Geometry check sheet. Reference: the model listing, model coordinates, mm. Face numbers are marked on the shaded views. A direction names the side the tool comes from. Round coordinates to 2 decimals unless told otherwise and drop trailing zeros. Order: outer loops, then holes, each group sorted by start corner. A loop starts at its lowest first (then second) coordinate and runs counter-clockwise, first axis right, second up. Notation, with made-up numbers: (22, -39) -> (54, -39) arc R22 ccw to (54, -14) -> close; hole circle Ø1 at (-8.75, 18.25). An arc over 180 degrees is marked (long way). Use a Markdown table: item, result. Add a question column.
Item 1: Set-up check for the marked faces 4 and 5: record each of +Z, -Z, +X, -X, +Y, -Y from which the full face is reachable in a straight line by a thin tool's end or side.
Item 2: Sectioned sample at A-A, the plane z = 0. Record the cut outline in (x, y).
Item 3: Sectioned sample at D-D, the plane z = 17. Record the cut outline in (x, y), and give its area (3 significant figures).
Item 4: Material ranges on probe 1 along X at (y, z) = (9.25, 0); probe 2 along Y at (x, z) = (24, 14); probe 3 along Y at (x, z) = (16, 2.5), recorded low to high. Write a range as [from, to].
Item 5: Sectioned sample at B-B, the plane x = 20. Record the cut outline in (y, z).
Item 6: Mould release check, pull along Z, two halves, no side actions. Record for the marked faces 1, 2 and 3: pulls with the +Z half, pulls with the -Z half, needs draft (parallel to the pull), parting line crosses it, or undercut.
Item 7: Gauge pin test, flat ends, axial feed: pin 1 Ø5 at (x, z) = (22.5, -1.5) entering from +Y; pin 2 Ø6 at (x, z) = (20, 0) entering from +Y. Record the tip position at first contact, or that the pin passes through.
Item 8: Sectioned sample at C-C, the plane y = 26. Record the cut outline in (x, z), and give its area (3 significant figures).
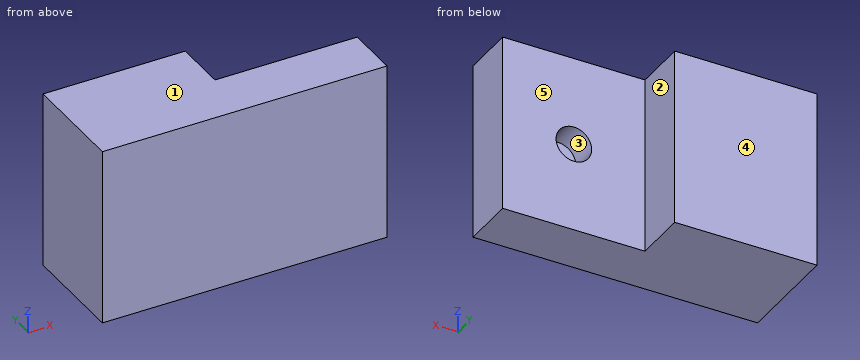
from build123d import *

# Parameters (mm, degrees)
EXTRUDE_START       = -25
EXTRUDE_1_DEPTH     = 50
SKETCH_2_R          = 5
CUT_EXTRUDE_1_DEPTH = 8


# Read off the part's stored shape, not the designer's step: 凸台-拉伸1
with BuildPart() as part:
    # 凸台-拉伸1 outline → 凸台-拉伸1 (new body)
    with BuildSketch(Plane.XY.offset(EXTRUDE_START)):
        Polygon((-40, 30), (-40, 0), (40, 0), (40, 15), (0, 15), (0, 30), align=None)
    extrude(amount=EXTRUDE_1_DEPTH)

    # 草图2 → 切除-拉伸1 (cut)
    with BuildSketch(Plane(origin=(0, 15, 0), x_dir=(1, 0, 0), z_dir=(0, 1, 0))):
        with Locations(Location((20, 0, 0), (0, 0, 270))):
            Circle(SKETCH_2_R)
    extrude(amount=-CUT_EXTRUDE_1_DEPTH, mode=Mode.SUBTRACT)


solid = part.part
Found:
| question | item | result |
|---|---|---|
| 1 | face 4 | +Z, -Z, +X, -X, +Y |
| 1 | face 5 | +Z, -Z, +X, +Y |
| 2 | outline | (-40, 0) -> (40, 0) -> (40, 15) -> (25, 15) -> (25, 7) -> (15, 7) -> (15, 15) -> (0, 15) -> (0, 30) -> (-40, 30) -> close |
| 3 | outline | (-40, 0) -> (40, 0) -> (40, 15) -> (0, 15) -> (0, 30) -> (-40, 30) -> close |
| 3 | area | 1,800 mm2 |
| 4 | probe 1 | x = [-40, 15], [25, 40] |
| 4 | probe 2 | y = [0, 15] |
| 4 | probe 3 | y = [0, 7] |
| 5 | outline | (0, -25) -> (15, -25) -> (15, -5) -> (7, -5) -> (7, 5) -> (15, 5) -> (15, 25) -> (0, 25) -> close |
| 6 | face 1 | pulls with the +Z half |
| 6 | face 2 | needs draft |
| 6 | face 3 | undercut |
| 7 | pin 1 | stops at y = 15 |
| 7 | pin 2 | stops at y = 7 |
| 8 | outline | (-40, -25) -> (0, -25) -> (0, 25) -> (-40, 25) -> close |
| 8 | area | 2,000 mm2 |
